Verification items for the finished model (mm, model axes). A direction names the side the tool comes from. Give positions to 0.01 mm unless a question says otherwise; leave off trailing zeros. Write each loop counter-clockwise with the first axis right and the second up, starting at its lowest first coordinate (ties: lowest second). Pieces come first, ordered by that corner, then holes. Notation, with made-up numbers: (-38, -26.5) -> (11, -26.5) arc R23 cw to (11, -3.5) -> close; hole circle Ø2 at (48.5, 59.5). An arc over 180 degrees is marked (long way). Answer as CSV lines item,"result".
```python
from build123d import *

# Parameters (mm, degrees)
SKETCH1_W               = 165.1
SKETCH1_H               = 101.6
BOSS_EXTRUDE1_DEPTH     = 1.47955
F_1_4_CLEARANCE_HOLE1_D = 6.5278
F_4_CLEARANCE_HOLE1_D   = 2.9464


with BuildPart() as part:
    # Sketch1 → Boss-Extrude1 (new body, symmetric)
    with BuildSketch(Plane.XY):
        Rectangle(SKETCH1_W, SKETCH1_H)
        with BuildLine():
            ThreePointArc((-7.575, 15.3), (-4.4, 18.475), (-7.575, 21.65))
            Line((-7.575, 21.65), (-39.325, 21.65))
            ThreePointArc((-39.325, 21.65), (-42.5, 18.475), (-39.325, 15.3))
            Line((-39.325, 15.3), (-7.575, 15.3))
        make_face(mode=Mode.SUBTRACT)
    extrude(amount=BOSS_EXTRUDE1_DEPTH, both=True)

    # 1/4 Clearance Hole1 (through all)
    with Locations(Plane(origin=(-54.280585756, -28.309576901, 1.47955), x_dir=(1, 0, 0), z_dir=(0, 0, 1))):
        with Locations((-15.569414244, 66.409576901), (124.130585756, 66.409576901), (54.280585756, 66.409576901)):
            Hole(F_1_4_CLEARANCE_HOLE1_D / 2)

    # #4 Clearance Hole1 (through all)
    with Locations(Plane(origin=(-67.931660522, 13.630291587, 1.47955), x_dir=(1, 0, 0), z_dir=(0, 0, 1))):
        with Locations((105.931660522, -10.330291587), (51.321660522, -35.984291587), (-8.268339478, -58.080291587), (144.131660522, -58.080291587), (67.931660522, -58.080291587)):
            Hole(F_4_CLEARANCE_HOLE1_D / 2)


solid = part.part
```
1) Section check C-C (z = -0.05). State how many separate pieces and enclosed holes the cut face has, and give its area (3 significant figures).
Reported:
separate pieces,"1"
enclosed holes,"9"
area,"16,400 mm²"
2) Draft check along Y on faces 3 (the flat face through (-24, 15.3, 0)), 4 (the flat face through (-82.55, -1, 0)), 5 (the flat face through (-1, -50.8, 0)). Enter one of: +Y half, -Y half, draft (parallel to the pull), parting line (faces both ways), or undercut.
Reported:
face 3,"undercut"
face 4,"draft"
face 5,"-Y half"
3) Depth check by flat-ended pin: pin 1 (2.5 mm diameter, centred on x = 38, y = 3.3, fed in from +Z). Enter the tip coordinate at first touch or a pass-through.
Reported:
pin 1,"through"
4) Tool access check on faces 1 (the flat face through (-23, 21.65, 0)), 2 (the flat face through (-1, 1, 1.48)). Record the directions out of +Z, -Z, +X, -X, +Y, -Y that give a thin tool (end or side, any length) a straight path to the whole face; none if there is none.
Reported:
face 1,"+Z, -Z"
face 2,"+Z, +X, -X, +Y, -Y"
5) Section check A-A (x = -69.85). Record the boundary of the cut face in (y, z), and give its area (3 significant figures).
Reported:
outline,"(-50.8, -1.48) -> (34.84, -1.48) -> (34.84, 1.48) -> (-50.8, 1.48) -> close; (41.36, -1.48) -> (50.8, -1.48) -> (50.8, 1.48) -> (41.36, 1.48) -> close"
area,"281 mm²"
6) Section check B-B (y = 17.5). Record the boundary of the cut face in (x, z).
Reported:
outline,"(-82.55, -1.48) -> (-42.35, -1.48) -> (-42.35, 1.48) -> (-82.55, 1.48) -> close; (-4.55, -1.48) -> (82.55, -1.48) -> (82.55, 1.48) -> (-4.55, 1.48) -> close"
7) Scan lines: line 1 along X through (y, z) = (38, 0.75); line 2 along Y through (x, z) = (-19.5, -1); line 3 along X through (y, z) = (40, -1). Record each from-to range of solid material in increasing order.
Reported:
line 1,"-82.55 to -73.11, -66.59 to -3.26, 3.26 to 66.59, 73.11 to 82.55"
line 2,"-50.8 to 15.3, 21.65 to 50.8"
line 3,"-82.55 to -72.5, -67.2 to -2.65, 2.65 to 67.2, 72.5 to 82.55"
